Design review of the part built by this model. Coordinates are the model's own, in mm. Give positions to 0.01 mm unless a question says otherwise; leave off trailing zeros. Loops run counter-clockwise (first coordinate to the right, second up) from the corner with the lowest first, then second, coordinate; pieces in that order, holes last. Notation, with made-up numbers: (-7, 68.5) - (25, 68.5) arc R18 cw to (25, 96.5) - close; hole circle Ø2 at (24, 74). An arc over 180 degrees is marked (long way). Put each result on its own line as item: value. Start each with the question number.
```python
from build123d import *

# Parameters (mm, degrees)
AUFSATZ_LINEAR_AUSTRAGEN1_DEPTH = 4
SCHNITT_LINEAR_AUSTRAGEN1_REACH = 6
SKIZZE2_R                       = 8
SKIZZE2_R_2                     = 2.141321697
SCHNITT_LINEAR_START            = -4
SCHNITT_LINEAR_AUSTRAGEN2_DEPTH = 4
AUFSATZ_LINEAR_AUSTRAGEN3_DEPTH = 4
SCHNITT_LINEAR_AUSTRAGEN3_REACH = 6
SKIZZE5_W                       = 3.5
SKIZZE5_H                       = 12
AUFSATZ_LINEAR_AUSTRAGEN4_DEPTH = 4
SKIZZE7_R                       = 1.55
SCHNITT_LINEAR_AUSTRAGEN4_DEPTH = 10


with BuildPart() as part:
    # Skizze1 → Aufsatz-Linear austragen1 (new body)
    with BuildSketch(Plane.XY):
        with BuildLine():
            Line((8.570550732, -10.430515814), (-71.429449268, -10.430515814))
            ThreePointArc((-71.429449268, -10.430515814), (-93.5, 0), (-71.429449268, 10.430515814))
            Line((-71.429449268, 10.430515814), (-65.575289804, 10.430515814))
            ThreePointArc((-65.575289804, 10.430515814), (-61.49939442, 6.35462043), (-57.423499036, 10.430515814))
            Line((-57.423499036, 10.430515814), (8.570550732, 10.430515814))
            ThreePointArc((8.570550732, 10.430515814), (19.001066546, 0), (8.570550732, -10.430515814))
        make_face()
    extrude(amount=AUFSATZ_LINEAR_AUSTRAGEN1_DEPTH)

    # Skizze2 → Schnitt-Linear austragen1 (cut, up to next)
    with BuildSketch(Plane.XY.offset(4), mode=Mode.PRIVATE) as schnitt_linear_austragen1_sk1:
        with Locations((-80, 0)):
            Circle(SKIZZE2_R)
    schnitt_linear_austragen1_tool1 = extrude(schnitt_linear_austragen1_sk1.sketch, amount=-SCHNITT_LINEAR_AUSTRAGEN1_REACH, mode=Mode.PRIVATE) & part.part
    add(schnitt_linear_austragen1_tool1.solids().sort_by_distance((-80, 0, 4))[0], mode=Mode.SUBTRACT)
    # Skizze2 → Schnitt-Linear austragen1 (cut, up to next)
    with BuildSketch(Plane.XY.offset(4), mode=Mode.PRIVATE) as schnitt_linear_austragen1_sk2:
        with Locations((-56.152824314, 1.105869461)):
            Circle(SKIZZE2_R_2)
    schnitt_linear_austragen1_tool2 = extrude(schnitt_linear_austragen1_sk2.sketch, amount=-SCHNITT_LINEAR_AUSTRAGEN1_REACH, mode=Mode.PRIVATE) & part.part
    add(schnitt_linear_austragen1_tool2.solids().sort_by_distance((-56.152824, 1.105869, 4))[0], mode=Mode.SUBTRACT)
    # Skizze2 → Schnitt-Linear austragen1 (cut, up to next)
    with BuildSketch(Plane.XY.offset(4), mode=Mode.PRIVATE) as schnitt_linear_austragen1_sk3:
        Polygon((-5.196152423, 4.033585801), (0, 7.033585801), (2, 3.569484186), (-3.196152423, 0.569484186), align=None)
    schnitt_linear_austragen1_tool3 = extrude(schnitt_linear_austragen1_sk3.sketch, amount=-SCHNITT_LINEAR_AUSTRAGEN1_REACH, mode=Mode.PRIVATE) & part.part
    add(schnitt_linear_austragen1_tool3.solids().sort_by_distance((-1.598076, 3.801535, 4))[0], mode=Mode.SUBTRACT)

    # Skizze3 → Schnitt-Linear austragen2 (cut)
    with BuildSketch(Plane.XY.offset(4).offset(SCHNITT_LINEAR_START)):
        Polygon((12.98673942, 30.628285162), (33.019811303, -4.070013171), (4.402698179, -20.592111136), (-2.330127019, -8.930515814), (8.92820323, -2.430515814), (-1.07179677, 14.889992262), (-12.330127019, 8.389992262), (-15.630373703, 14.106187196), align=None)
    extrude(amount=SCHNITT_LINEAR_AUSTRAGEN2_DEPTH, mode=Mode.SUBTRACT)

    # Skizze4 → Aufsatz-Linear austragen3 (add)
    with BuildSketch(Plane.XY):
        with BuildLine():
            Line((-8.795836552, 10.430515814), (-1.07179677, 14.889992262))
            ThreePointArc((-1.07179677, 14.889992262), (0.435735022, 15.092552947), (1.649755119, 14.176126114))
            Line((1.649755119, 14.176126114), (9.66025479, 0.301533691))
            ThreePointArc((9.66025479, 0.301533691), (9.860054688, -1.216103823), (8.92820323, -2.430515814))
            Line((8.92820323, -2.430515814), (1.502883158, 10.430515814))
            Line((1.502883158, 10.430515814), (-8.795836552, 10.430515814))
        make_face()
    extrude(amount=AUFSATZ_LINEAR_AUSTRAGEN3_DEPTH)

    # Skizze5 → Schnitt-Linear austragen3 (cut, up to next)
    with BuildSketch(Plane.XY.offset(4), mode=Mode.PRIVATE) as schnitt_linear_austragen3_sk1:
        with Locations((-35.258223841, 0)):
            Rectangle(SKIZZE5_W, SKIZZE5_H)
    schnitt_linear_austragen3_tool1 = extrude(schnitt_linear_austragen3_sk1.sketch, amount=-SCHNITT_LINEAR_AUSTRAGEN3_REACH, mode=Mode.PRIVATE) & part.part
    add(schnitt_linear_austragen3_tool1.solids().sort_by_distance((-35.258224, 0, 4))[0], mode=Mode.SUBTRACT)

    # Skizze6 → Aufsatz-Linear austragen4 (add)
    with BuildSketch(Plane.XY.offset(4)):
        with BuildLine():
            Line((-63.811678178, -10.430515814), (-53.840299994, -10.430515814))
            ThreePointArc((-53.840299994, -10.430515814), (-58.825989086, -15.808542635), (-63.811678178, -10.430515814))
        make_face()
    extrude(amount=-AUFSATZ_LINEAR_AUSTRAGEN4_DEPTH)

    # Skizze7 → Schnitt-Linear austragen4 (cut)
    with BuildSketch(Plane.XY.offset(4)):
        with Locations((-58.659847502, -12.012547734)):
            Circle(SKIZZE7_R)
        with Locations((-43.4, -3.025056359)):
            Circle(SKIZZE7_R)
    extrude(amount=-SCHNITT_LINEAR_AUSTRAGEN4_DEPTH, mode=Mode.SUBTRACT)


solid = part.part
```
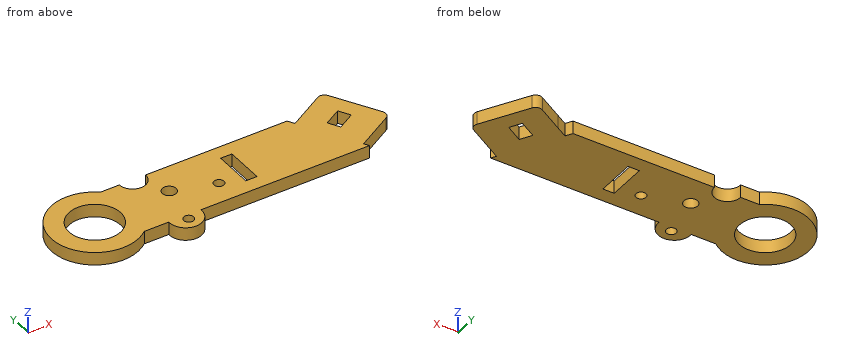
Item 1: Consider section B-B (z = 1.45). State the section outline as (x, y) points, plus the area to 3 significant figures.
Item 2: Consider section D-D (x = -20). State the section outline as (y, z) points.
Item 3: For L1, parallel to X at y = -2, z = 1.65; L2, parallel to Y at x = -43.4, z = 1.45; L3, parallel to X at y = -11, z = 1.85, list the stretches that pass through material, from the lowest coordinate up. Write a range as from..to.
Item 4: Consider section A-A (x = -35.5). State the section outline as (y, z) points, plus the area to 3 significant figures.
Item 5: Consider section C-C (y = 2). State the section outline as (x, z) points, plus the area to 3 significant figures.
Item 6: For P1, Ø1.8, axis at x = -35.5, z = 1.5, coming from the -Y side; P2, Ø1.5, axis at x = -76.5, z = 2.5, coming from the +Y side; P3, Ø1.2, axis at x = -32.5, z = 2.5, coming from the +Y side; P4, Ø3, axis at x = -58.66, y = -12.01, coming from the -Z side, all flat-tipped, find the tip position at first contact; note any pin that passes through.
Geometry says:
1. outline: (-71.43, -10.43) - (-63.81, -10.43) arc R5 ccw (long way) to (-53.84, -10.43) - (-1.46, -10.43) - (-2.33, -8.93) - (8.93, -2.43) arc R2 ccw to (9.66, 0.3) - (1.65, 14.18) arc R2 ccw to (-1.07, 14.89) - (-12.33, 8.39) - (-13.51, 10.43) - (-57.42, 10.43) arc R4.08 cw to (-65.58, 10.43) - (-71.43, 10.43) arc R13.5 ccw (long way) to start; hole circle Ø16 at (-80, 0); hole circle Ø3.1 at (-58.66, -12.01); hole circle Ø4.28 at (-56.15, 1.11); hole circle Ø3.1 at (-43.4, -3.03); hole (-37.01, -6) - (-33.51, -6) - (-33.51, 6) - (-37.01, 6) - close; hole (-5.2, 4.03) - (-3.2, 0.57) - (2, 3.57) - (0, 7.03) - close
1. area: 1,850 mm2
2. outline: (-10.43, 0) - (10.43, 0) - (10.43, 4) - (-10.43, 4) - close
3. L1: x = -93.35..-87.75, -72.25..-44.56, -42.24..-37.01, -33.51..9.45
3. L2: y = -10.43..-4.58, -1.48..10.43
3. L3: x = -87.83..-72.17, -63.82..-59.83, -57.49..-53.83
4. outline: (-10.43, 0) - (-6, 0) - (-6, 4) - (-10.43, 4) - close; (6, 0) - (10.43, 0) - (10.43, 4) - (6, 4) - close
4. area: 35.4 mm2
5. outline: (-93.35, 0) - (-87.75, 0) - (-87.75, 4) - (-93.35, 4) - close; (-72.25, 0) - (-58.1, 0) - (-58.1, 4) - (-72.25, 4) - close; (-54.21, 0) - (-37.01, 0) - (-37.01, 4) - (-54.21, 4) - close; (-33.51, 0) - (-4.02, 0) - (-4.02, 4) - (-33.51, 4) - close; (-0.72, 0) - (8.68, 0) - (8.68, 4) - (-0.72, 4) - close
5. area: 303 mm2
6. P1: stops at y = -10.43
6. P2: stops at y = 13.22
6. P3: stops at y = 10.43
6. P4: passes through
